Could you check a few things on this model? Use its own coordinates, in mm. A direction names the side the tool comes from. Round coordinates to 2 decimals unless told otherwise and drop trailing zeros. Loops run counter-clockwise (first coordinate to the right, second up) from the corner with the lowest first, then second, coordinate; pieces in that order, holes last. Notation, with made-up numbers: (23, 56.5) -> (75, 56.5) arc R27 cw to (75, 82.5) -> close; hole circle Ø4 at (69.25, -5.5). An arc over 180 degrees is marked (long way). One line per item, written item: value.
from build123d import *

# Parameters (mm, degrees)
SKETCH1_R                = 2.55
BOSS_EXTRUDE1_DEPTH      = 5
SKETCH4_R                = 4.5
CUT_EXTRUDE2_DEPTH       = 1
SKETCH6_W                = 5.947651005
SKETCH6_H                = 20
BOSS_EXTRUDE2_DEPTH      = 4
BOSS_EXTRUDE2_DEPTH_BACK = 4
SKETCH11_R               = 4.5
CUT_EXTRUDE3_DEPTH       = 0.5
SKETCH16_R               = 3.25
SKETCH16_R_2             = 2.5
BOSS_EXTRUDE3_DEPTH      = 3
BOSS_EXTRUDE3_DEPTH_BACK = 3
FILLET3_R                = 2
BOSS_EXTRUDE4_DEPTH      = 5.947651
CUT_EXTRUDE5_REACH       = 85
SKETCH18_R               = 3.25
SKETCH18_R_2             = 2.5


with BuildPart() as part:
    # Sketch1 → Boss-Extrude1 (new body)
    with BuildSketch(Plane.XY):
        with BuildLine():
            Line((100, 25), (100, 20))
            ThreePointArc((100, 20), (99.414213562, 18.585786438), (98, 18))
            Line((98, 18), (72.248595461, 18))
            ThreePointArc((72.248595461, 18), (71.130561473, 17.658312395), (70.39454584, 16.75))
            ThreePointArc((70.39454584, 16.75), (50, 3), (29.60545416, 16.75))
            ThreePointArc((29.60545416, 16.75), (28.869438527, 17.658312395), (27.751404539, 18))
            Line((27.751404539, 18), (2, 18))
            ThreePointArc((2, 18), (0.585786438, 18.585786438), (0, 20))
            Line((0, 20), (0, 25))
            Line((0, 25), (0, 30))
            ThreePointArc((0, 30), (0.585786438, 31.414213562), (2, 32))
            Line((2, 32), (21.056240945, 32))
            Line((21.056240945, 32), (27.751404539, 32))
            ThreePointArc((27.751404539, 32), (28.869438527, 32.341687605), (29.60545416, 33.25))
            ThreePointArc((29.60545416, 33.25), (30.166752838, 34.520625347), (30.807119991, 35.753295167))
            ThreePointArc((30.807119991, 35.753295167), (32.106461975, 36.725482012), (33.699080137, 36.414026968))
            Line((33.699080137, 36.414026968), (35.34656276, 35.260447216))
            ThreePointArc((35.34656276, 35.260447216), (36.146649881, 34.078494315), (35.955031011, 32.664127224))
            ThreePointArc((35.955031011, 32.664127224), (50, 9), (64.044968989, 32.664127224))
            ThreePointArc((64.044968989, 32.664127224), (63.853350119, 34.078494315), (64.65343724, 35.260447216))
            Line((64.65343724, 35.260447216), (66.300919863, 36.414026968))
            ThreePointArc((66.300919863, 36.414026968), (67.893538025, 36.725482012), (69.192880009, 35.753295167))
            ThreePointArc((69.192880009, 35.753295167), (69.833247162, 34.520625347), (70.39454584, 33.25))
            ThreePointArc((70.39454584, 33.25), (71.130561473, 32.341687605), (72.248595461, 32))
            Line((72.248595461, 32), (78.943759055, 32))
            Line((78.943759055, 32), (98, 32))
            ThreePointArc((98, 32), (99.414213562, 31.414213562), (100, 30))
            Line((100, 30), (100, 25))
        make_face()
        with Locations((93, 25)):
            Circle(SKETCH1_R, mode=Mode.SUBTRACT)
        with Locations((7, 25)):
            Circle(SKETCH1_R, mode=Mode.SUBTRACT)
    extrude(amount=BOSS_EXTRUDE1_DEPTH)

    # Sketch4 → Cut-Extrude2 (cut)
    with BuildSketch(Plane.XY.offset(5)):
        with Locations((93, 25)):
            Circle(SKETCH4_R)
        with Locations((7, 25)):
            Circle(SKETCH4_R)
    extrude(amount=-CUT_EXTRUDE2_DEPTH, mode=Mode.SUBTRACT)

    # Sketch6 → Boss-Extrude2 (add, two sides)
    with BuildSketch(Plane(origin=(0, 25, 0), x_dir=(-1, 0, 0), z_dir=(0, -1, 0))) as boss_extrude2_sk:
        with Locations((-80.026174497, -15)):
            Rectangle(SKETCH6_W, SKETCH6_H)
    extrude(amount=BOSS_EXTRUDE2_DEPTH)
    extrude(boss_extrude2_sk.sketch, amount=-BOSS_EXTRUDE2_DEPTH_BACK)

    # Sketch11 → Cut-Extrude3 (cut)
    with BuildSketch(Plane(origin=(0, 0, 0), x_dir=(-1, 0, 0), z_dir=(0, 0, -1))):
        with Locations((-93, 25)):
            Circle(SKETCH11_R)
        with Locations((-7, 25)):
            Circle(SKETCH11_R)
    extrude(amount=-CUT_EXTRUDE3_DEPTH, mode=Mode.SUBTRACT)

    # Sketch16 → Boss-Extrude3 (add, two sides)
    with BuildSketch(Plane(origin=(0, 25, 0), x_dir=(-1, 0, 0), z_dir=(0, -1, 0))) as boss_extrude3_sk:
        with BuildLine():
            Line((-30.494270905, -5), (-22.494270905, -5))
            Line((-22.494270905, -5), (-22.494270905, -71))
            ThreePointArc((-22.494270905, -71), (-23.665843781, -73.828427125), (-26.494270905, -75))
            Line((-26.494270905, -75), (-30.494270905, -75))
            Line((-30.494270905, -75), (-47.361403242, -75))
            ThreePointArc((-47.361403242, -75), (-57.917236977, -76.464101615), (-53.018257491, -67))
            Line((-53.018257491, -67), (-34.494270905, -67))
            ThreePointArc((-34.494270905, -67), (-31.665843781, -65.828427125), (-30.494270905, -63))
            Line((-30.494270905, -63), (-30.494270905, -60.732138804))
            Line((-30.494270905, -60.732138804), (-47.361403242, -60.732138804))
            ThreePointArc((-47.361403242, -60.732138804), (-57.917236977, -62.196240419), (-53.018257491, -52.732138804))
            Line((-53.018257491, -52.732138804), (-34.494270905, -52.732138804))
            ThreePointArc((-34.494270905, -52.732138804), (-31.665843781, -51.560565928), (-30.494270905, -48.732138804))
            Line((-30.494270905, -48.732138804), (-30.494270905, -5))
        make_face()
        with Locations((-53.018257491, -73)):
            Circle(SKETCH16_R, mode=Mode.SUBTRACT)
        with Locations((-53.018257491, -58.732138804)):
            Circle(SKETCH16_R_2, mode=Mode.SUBTRACT)
    extrude(amount=BOSS_EXTRUDE3_DEPTH)
    extrude(boss_extrude3_sk.sketch, amount=-BOSS_EXTRUDE3_DEPTH_BACK)

    # Fillet3
    fillet3_edges = [part.edges().sort_by_distance(p)[0] for p in [
        (83, 25, 5),
        (80.026174498, 29, 5),
        (77.052348995, 25, 5),
        (80.026174498, 21, 5),
        (30.494270905, 25, 5),
        (26.494270905, 28, 5),
        (22.494270905, 25, 5),
        (26.494270905, 22, 5),
    ]]
    fillet(fillet3_edges, radius=FILLET3_R)

    # Sketch17 → Boss-Extrude4 (add)
    with BuildSketch(Plane(origin=(83, 0, 0), x_dir=(0, 0, -1), z_dir=(1, 0, 0))):
        with BuildLine():
            ThreePointArc((-19.547210182, 27.503414308), (-31, 25), (-19.547210182, 22.496585692))
            ThreePointArc((-19.547210182, 22.496585692), (-8.094420363, 25), (-19.547210182, 27.503414308))
        make_face()
    extrude(amount=-BOSS_EXTRUDE4_DEPTH)

    # Sketch18 → Cut-Extrude5 (cut, up to next)
    with BuildSketch(Plane(origin=(83, 0, 0), x_dir=(0, 0, -1), z_dir=(1, 0, 0)), mode=Mode.PRIVATE) as cut_extrude5_sk1:
        with Locations((-25, 25)):
            Circle(SKETCH18_R)
    cut_extrude5_tool1 = extrude(cut_extrude5_sk1.sketch, amount=-CUT_EXTRUDE5_REACH, mode=Mode.PRIVATE) & part.part
    add(cut_extrude5_tool1.solids().sort_by_distance((83, 25, 25))[0], mode=Mode.SUBTRACT)
    # Sketch18 → Cut-Extrude5 (cut, up to next)
    with BuildSketch(Plane(origin=(83, 0, 0), x_dir=(0, 0, -1), z_dir=(1, 0, 0)), mode=Mode.PRIVATE) as cut_extrude5_sk2:
        with Locations((-14.094420363, 25)):
            Circle(SKETCH18_R_2)
    cut_extrude5_tool2 = extrude(cut_extrude5_sk2.sketch, amount=-CUT_EXTRUDE5_REACH, mode=Mode.PRIVATE) & part.part
    add(cut_extrude5_tool2.solids().sort_by_distance((83, 25, 14.09442))[0], mode=Mode.SUBTRACT)


solid = part.part
(1) If we section it at D-D, the plane z = 25: Please give me the cut outline in (x, y), then the cut area to 3 significant figures.
Recorded:
outline: (22.49, 22) -> (30.49, 22) -> (30.49, 28) -> (22.49, 28) -> close; (77.05, 19) -> (83, 19) -> (83, 21.75) -> (77.05, 21.75) -> close; (77.05, 28.25) -> (83, 28.25) -> (83, 31) -> (77.05, 31) -> close
area: 80.7 mm²
(2) If we section it at C-C, the plane y = 12.5: Please give me the cut outline in (x, z), then the cut area to 3 significant figures.
Recorded:
outline: (31.9, 0) -> (40.01, 0) -> (40.01, 5) -> (31.9, 5) -> close; (59.99, 0) -> (68.1, 0) -> (68.1, 5) -> (59.99, 5) -> close
area: 81.2 mm²
(3) For faces 1 (the face through (97.496, 25.198, 0.246)), 2 (the face through (36.14, 34.1, 2.46)), 3 (the face through (44, 25, 67)), which set-ups out of +Z, -Z, +X, -X, +Y, -Y let a thin tool reach every point of the face, with its end or its side?
Recorded:
face 1: -Z
face 2: +Z, -Z
face 3: +X, +Y, -Y
(4) I'm going to push flat-ended pins straight in: pin 1 Ø3 at (y, z) = (25.5, 25) entering from +X; pin 2 Ø6.5 at (x, y) = (47.5, 25.5) entering from -Z; pin 3 Ø8 at (x, z) = (21.5, 46) entering from +Y; pin 4 Ø12 at (x, y) = (52, 10.5) entering from -Z. Where does each tip first touch, or does it pass through?
Recorded:
pin 1: x = 30.49
pin 2: z = 52.73
pin 3: y = 28
pin 4: z = 0
(5) If we section it at A-A, the plane x = 93: Please give me the cut outline in (y, z), then the cut area to 4 significant figures.
Recorded:
outline: (18, 0) -> (20.5, 0) -> (20.5, 0.5) -> (22.45, 0.5) -> (22.45, 4) -> (20.5, 4) -> (20.5, 5) -> (18, 5) -> close; (27.55, 0.5) -> (29.5, 0.5) -> (29.5, 0) -> (32, 0) -> (32, 5) -> (29.5, 5) -> (29.5, 4) -> (27.55, 4) -> close
area: 38.65 mm²
(6) If I drill on L1, parallel to X at y = 25, z = 3; L2, parallel to X at y = 26.5, z = 11; L3, parallel to Y at x = 81.55, z = 25, over which ranges is the centre line in solid material (lowest first)?
Recorded:
L1: 0 to 4.45, 9.55 to 34, 66 to 90.45, 95.55 to 100
L2: 22.49 to 30.49, 77.05 to 83
L3: 19 to 21.75, 28.25 to 31
(7) Thinking about a two-plate mould opening in X: for faces 4 (the face through (80, 29, 8)), 5 (the face through (0.6, 18.57, 2.46)), 6 (the face through (31.7, 24.96, 65.86)), which applies, released by +X, released by -X, zero draft, split by the parting line, or undercut?
Recorded:
face 4: zero draft
face 5: released by -X
face 6: undercut
(8) If we section it at B-B, the plane z = 73: Please give me the cut outline in (x, y), then the cut area to 3 significant figures.
Recorded:
outline: (23.03, 22) -> (49.77, 22) -> (49.77, 28) -> (23.03, 28) -> close; (56.27, 22) -> (59.02, 22) -> (59.02, 28) -> (56.27, 28) -> close
area: 177 mm²
